Geometry: final body of the model. Coordinates: model frame, mm. A direction names the side the tool comes from. Round coordinates to 2 decimals unless told otherwise and drop trailing zeros. Loops run counter-clockwise (first coordinate to the right, second up) from the corner with the lowest first, then second, coordinate; pieces in that order, holes last. Notation, with made-up numbers: (31.25, 25.5) - (83.25, 25.5) arc R20 cw to (83.25, 60.5) - close; hole circle Ø8 at (19.5, -17.5). An arc over 180 degrees is marked (long way). Use CSV: the item, a comma, the result in double quotes.
from build123d import *

# Parameters (mm, degrees)
SKETCH_1_R          = 3.25
EXTRUDE_1_DEPTH     = 19.5
SKETCH_2_W          = 14
SKETCH_2_H          = 15
EXTRUDE_2_DEPTH     = 2
EXTRUDE_3_DEPTH     = 14
FILLET_1_R          = 2
SKETCH_5_W          = 24
SKETCH_5_H          = 25
EXTRUDE_4_DEPTH     = 20
SKETCH_6_W          = 2.5
SKETCH_6_H          = 2.5
CUT_EXTRUDE_1_DEPTH = 40.298536868
SKETCH_7_W          = 3
SKETCH_7_H          = 3
CUT_EXTRUDE_2_DEPTH = 39.226299847
SKETCH_8_W          = 8
SKETCH_8_H          = 9
CUT_EXTRUDE_3_DEPTH = 43.744151647
SKETCH_9_W          = 2.5
SKETCH_9_H          = 2.5
EXTRUDE_5_DEPTH     = 11.5
FILLET_7_R          = 12
EXTRUDE_6_DEPTH     = 5
EXTRUDE_START       = -5
EXTRUDE_7_DEPTH     = 5


with BuildPart() as part:
    # Sketch 1 → Extrude 1 (new body)
    with BuildSketch(Plane.XY):
        Circle(SKETCH_1_R)
    extrude(amount=EXTRUDE_1_DEPTH)



with BuildPart() as body_2:
    # Sketch 2 → Extrude 2 (new body)
    with BuildSketch(Plane(origin=(5, 0, 0), x_dir=(0, 0, -1), z_dir=(1, 0, 0))):
        with Locations((-9.75, 0)):
            Rectangle(SKETCH_2_W, SKETCH_2_H)
    extrude(amount=EXTRUDE_2_DEPTH)


with BuildPart() as part_1:
    add(part.part)

    add(body_2.part)  # Extrude 3 merges body 2
    # Sketch 3 → Extrude 3 (add)
    with BuildSketch(Plane(origin=(0, 0, 2.75), x_dir=(-1, 0, 0), z_dir=(0, 0, -1))):
        Polygon((0, 0), (-5, 4.5), (-5, -4.5), align=None)
    extrude(amount=-EXTRUDE_3_DEPTH)

    # Fillet 1
    fillet_1_edges = [part_1.edges().sort_by_distance(p)[0] for p in [
        (2.415705975, 2.174135378, 9.75),
        (2.415705975, -2.174135378, 9.75),
        (5, 4.5, 9.75),
        (5, -4.5, 9.75),
    ]]
    fillet(fillet_1_edges, radius=FILLET_1_R)

    # Sketch 5 → Extrude 4 (add)
    with BuildSketch(Plane(origin=(7, 0, 0), x_dir=(0, 0, -1), z_dir=(1, 0, 0))):
        with Locations((-9.75, 0)):
            Rectangle(SKETCH_5_W, SKETCH_5_H)
    extrude(amount=EXTRUDE_4_DEPTH)

    # Sketch 6 → Cut-Extrude 1 (cut, through all)
    with BuildSketch(Plane(origin=(27, 0, 0), x_dir=(0, 0, -1), z_dir=(1, 0, 0))):
        with Locations((-13, 0)):
            Rectangle(SKETCH_6_W, SKETCH_6_H)
        with Locations((-6.5, 0)):
            Rectangle(SKETCH_6_W, SKETCH_6_H)
    extrude(amount=-CUT_EXTRUDE_1_DEPTH, mode=Mode.SUBTRACT)

    # Sketch 7 → Cut-Extrude 2 (cut, through all)
    with BuildSketch(Plane.XY.offset(21.75)):
        with Locations((9, 0)):
            Rectangle(SKETCH_7_W, SKETCH_7_H)
        with Locations((14, 0)):
            Rectangle(SKETCH_7_W, SKETCH_7_H)
    extrude(amount=-CUT_EXTRUDE_2_DEPTH, mode=Mode.SUBTRACT)

    # Sketch 8 → Cut-Extrude 3 (cut, through all)
    with BuildSketch(Plane(origin=(0, 12.5, 0), x_dir=(1, 0, 0), z_dir=(0, 1, 0))):
        with Locations((11.5, -9.75)):
            Rectangle(SKETCH_8_W, SKETCH_8_H)
    extrude(amount=-CUT_EXTRUDE_3_DEPTH, mode=Mode.SUBTRACT)

    # Sketch 9 → Extrude 5 (add)
    with BuildSketch(Plane.ZY.offset(-15.5)):
        with Locations((13, 0)):
            Rectangle(SKETCH_9_W, SKETCH_9_H)
        with Locations((6.5, 0)):
            Rectangle(SKETCH_9_W, SKETCH_9_H)
    extrude(amount=-EXTRUDE_5_DEPTH)

    # Fillet 7
    # the kernel refuses this fillet: 12 mm, written as the material it takes off along each edge
    with BuildSketch(Plane(origin=(27, -12.5, 51.75), x_dir=(-1, 0, 0), z_dir=(0, 0, -1))) as fillet_7_piece_1:
        with BuildLine():
            CenterArc((FILLET_7_R, FILLET_7_R), FILLET_7_R, 180, 90)
            Line((0, FILLET_7_R), (0, 0))
            Line((0, 0), (FILLET_7_R, 0))
        make_face()
    extrude(amount=84, mode=Mode.SUBTRACT)
    with BuildSketch(Plane(origin=(27, 12.5, -32.25), x_dir=(0, -1, 0), z_dir=(0, 0, 1))) as fillet_7_piece_2:
        with BuildLine():
            CenterArc((FILLET_7_R, -FILLET_7_R), FILLET_7_R, 90, 90)
            Line((0, -FILLET_7_R), (0, 0))
            Line((0, 0), (FILLET_7_R, 0))
        make_face()
    extrude(amount=84, mode=Mode.SUBTRACT)

    # Sketch 10 → Extrude 6 (add)
    with BuildSketch(Plane(origin=(0, 0, 2.75), x_dir=(-1, 0, 0), z_dir=(0, 0, -1))):
        with BuildLine():
            Line((1.805058135, 5.248263058), (1.433861829, 10))
            Line((1.433861829, 10), (-7, 12.5))
            Line((-7, 12.5), (-7, -12.5))
            Line((-7, -12.5), (2.991476943, -9.939253626))
            Line((2.991476943, -9.939253626), (2.598155739, -4.904292687))
            ThreePointArc((2.598155739, -4.904292687), (-4.557007333, -3.167993713), (-3.692030902, 4.143839743))
            Line((-3.692030902, 4.143839743), (-4.42941418, 6.229991174))
            Line((-4.42941418, 6.229991174), (-0.469507268, 7.629683016))
            Line((-0.469507268, 7.629683016), (0.267876009, 5.543531586))
            ThreePointArc((0.267876009, 5.543531586), (1.046928779, 5.450361468), (1.805058135, 5.248263058))
        make_face()
    extrude(amount=EXTRUDE_6_DEPTH)

    # Sketch 11 → Extrude 7 (add)
    with BuildSketch(Plane(origin=(0, 0, 16.75), x_dir=(-1, 0, 0), z_dir=(0, 0, -1)).offset(EXTRUDE_START)):
        with BuildLine():
            Line((1.805058135, 5.248263058), (1.433861829, 10))
            Line((1.433861829, 10), (-7, 12.5))
            Line((-7, 12.5), (-7, -12.5))
            Line((-7, -12.5), (2.991476943, -9.939253626))
            Line((2.991476943, -9.939253626), (2.598155739, -4.904292687))
            ThreePointArc((2.598155739, -4.904292687), (-4.557007333, -3.167993713), (-3.692030902, 4.143839743))
            Line((-3.692030902, 4.143839743), (-4.42941418, 6.229991174))
            Line((-4.42941418, 6.229991174), (-0.469507268, 7.629683016))
            Line((-0.469507268, 7.629683016), (0.267876009, 5.543531586))
            ThreePointArc((0.267876009, 5.543531586), (1.046928779, 5.450361468), (1.805058135, 5.248263058))
        make_face()
    extrude(amount=EXTRUDE_7_DEPTH)


solid = part_1.part
Item 1: Section C-C on z = 10.75. Return the cut outline in (x, y), plus the area to 3 significant figures.
Final values:
outline,"(1.41, -2.93) arc R2 cw to (3.61, -3.25) - (4.34, -3.9) arc R2 cw to (5, -5.39) - (5, -7.5) - (7, -7.5) - (7, -12.5) - (7.5, -12.5) - (7.5, 12.5) - (7, 12.5) - (7, 7.5) - (5, 7.5) - (5, 5.39) arc R2 cw to (4.34, 3.9) - (3.61, 3.25) arc R2 cw to (1.41, 2.93) arc R3.25 ccw (long way) to start; (15.5, -12.49) arc R12 ccw to (27, -0.5) - (27, 0.5) arc R12 ccw to (15.5, 12.49) - close"
area,"317 mm²"
Item 2: Pin query (flat end, axial travel): P1, Ø10, axis at y = -6, z = 7, coming from the +X side; P2, Ø2, axis at x = 20.5, z = 8, coming from the +Y side; P3, Ø0.8, axis at x = 1, z = 6, coming from the -Y side. Return the tip coordinate at first contact, or that it passes through.
Final values:
P1,"stops at x = 26.99"
P2,"stops at y = 11.62"
P3,"stops at y = -3.19"
Item 3: Section A-A on y = 0. Give the number of separate pieces and of enclosed holes in the cut face, plus the area to 3 significant figures.
Final values:
separate pieces,"6"
enclosed holes,"0"
area,"458 mm²"
Item 4: Material intervals for line 1 (X direction, y = 0, z = 14.5); line 2 (Z direction, x = 1, y = 1); line 3 (Z direction, x = 2, y = -10), sorted ascending.
Final values:
line 1,"x = -3.25 to 7.5, 10.5 to 12.5, 15.5 to 27"
line 2,"z = 0 to 5.25, 7.75 to 11.75, 14.25 to 19.5"
line 3,"z = -2.25 to 2.75, 16.75 to 21.75"
Item 5: Section B-B on x = 14. Return the cut outline in (y, z).
Final values:
outline,"(-12.5, -2.25) - (-1.5, -2.25) - (-1.5, 5.25) - (-12.5, 5.25) - close; (-12.5, 14.25) - (-1.5, 14.25) - (-1.5, 21.75) - (-12.5, 21.75) - close; (1.5, -2.25) - (12.5, -2.25) - (12.5, 5.25) - (1.5, 5.25) - close; (1.5, 14.25) - (12.5, 14.25) - (12.5, 21.75) - (1.5, 21.75) - close"
Item 6: Reachability of faces 4 (the flat face through (2, 0, 14.25)), 5 (the flat face through (11, 0, 14.25)), 6 (the cylindrical face through (4.49, -3.26, 19.28)) from +Z, -Z, +X, -X, +Y, -Y: full face, straight path, thin tool, end or side. Return the list, or none.
Final values:
face 4,"-X"
face 5,"+Y, -Y"
face 6,"+Z"
Item 7: Mould query, pull axis Z, two halves, no side actions, for faces 1 (the cylindrical face through (2.571, 2.757, 9.652)), 2 (the flat face through (4, 0, 16.75)), 3 (the flat face through (5, 6, 10)). Classes: released by +Z, released by -Z, zero draft, split by the parting line, or undercut.
Final values:
face 1,"zero draft"
face 2,"released by +Z"
face 3,"undercut"
Item 8: Section D-D on y = 8. Return the cut outline in (x, z), plus the area to 3 significant figures.
Final values:
outline,"(-1.59, -2.25) - (24.37, -2.25) - (24.37, 21.75) - (-1.59, 21.75) - (-1.59, 16.75) - (7, 16.75) - (7, 2.75) - (-1.59, 2.75) - close; hole (7.5, 5.25) - (15.5, 5.25) - (15.5, 14.25) - (7.5, 14.25) - close"
area,"431 mm²"
